Part model, mm, in its own coordinate system. A direction names the side the tool comes from. Round coordinates to 2 decimals unless told otherwise and drop trailing zeros. Write each loop counter-clockwise with the first axis right and the second up, starting at its lowest first coordinate (ties: lowest second). Pieces come first, ordered by that corner, then holes. Notation, with made-up numbers: M -20,41 L -11,41 A24 cw -11,74 Z; hole C 56,42.5 d1. An arc over 180 degrees is marked long. Answer as a JSON object with one key per item and string values. Group by question number.
1. Which spindle directions (+Z, -Z, +X, -X, +Y, -Y) get a long thin tool onto all of the face, cutting with end or side? Do faces 5 (the face through (3.631, 11.381, -16.235)), 6 (the face through (49.75, 2.6, -28.5)), 7 (the face through (53.76, 18.983, -40.521)), 8 (the face through (9.31, 18.15, -2.18)), 9 (the face through (29, 10, -7.62)). Say none if no direction does.
2. Drill centre lines: line 1 (Y direction, x = 53.5, z = -40.6); line 2 (X direction, y = 1.75, z = -35.5). Where is each one in solid material? Low to high. Write a range as from..to.
3. Band-saw the part on A-A, the plane z = -25. Write the cut outline in (x, y).
4. Two-plate mould, pull along Z, no slides. Class faces 1 (the face through (29, 10, -10.2)), 2 (the face through (4, 12, -39)), 3 (the face through (29, 3.65, -4)), 4 (the face through (4, 3, -31)): +Z half, -Z half, draft (parallel to the pull), parting line (faces both ways), or undercut.
5. Band-saw the part on C-C, the plane x = 53.5. Write the cut outline in (y, z), plus the area to 3 significant figures.
6. Band-saw the part on D-D, the plane y = 7. Write the cut outline in (x, z).
7. Drop flat-ended pins along their axis: pin 1 (1.5 mm diameter, centred on x = 46.5, y = 14.5, fed in from +Z); pin 2 (10 mm diameter, centred on x = 45, y = 12.5, fed in from -Z); pin 3 (6 mm diameter, centred on x = 35.5, y = 7.5, fed in from -Z); pin 4 (6 mm diameter, centred on x = 2.5, z = -32.5, fed in from +Y). Give the stop position or say it passes through.
8. Band-saw the part on B-B, the plane y = 9.75. Write the cut outline in (x, z), plus the area to 3 significant figures.
from build123d import *

# Parameters (mm, degrees)
SKETCH1_W                 = 57.5
SKETCH1_H                 = 42
BOSS_EXTRUDE1_DEPTH       = 20
CUT_EXTRUDE1_DEPTH        = 21
CUT_EXTRUDE2_DEPTH        = 58.5
CUT_EXTRUDE3_REACH        = 44
SKETCH4_R                 = 2
SKETCH5_W                 = 7.62
SKETCH5_H                 = 12.7
CUT_EXTRUDE4_DEPTH        = 58.5
M4X0_7_TAPPED_HOLE1_D     = 3.3
M4X0_7_TAPPED_HOLE1_DEPTH = 3.65
CHAMFER1_SIZE             = 3


with BuildPart() as part:
    # Sketch1 → Boss-Extrude1 (new body)
    with BuildSketch(Plane(origin=(0, 0, 0), x_dir=(1, 0, 0), z_dir=(0, 1, 0))):
        with Locations((28.75, 21)):
            Rectangle(SKETCH1_W, SKETCH1_H)
    extrude(amount=BOSS_EXTRUDE1_DEPTH)

    # Sketch2 → Cut-Extrude1 (cut, through all)
    with BuildSketch(Plane(origin=(0, 20, 0), x_dir=(1, 0, 0), z_dir=(0, 1, 0))):
        with BuildLine():
            Line((7.75, 42), (7.75, 15.2))
            ThreePointArc((7.75, 15.2), (9.214466094, 11.664466094), (12.75, 10.2))
            Line((12.75, 10.2), (44.75, 10.2))
            ThreePointArc((44.75, 10.2), (48.285533906, 11.664466094), (49.75, 15.2))
            Line((49.75, 15.2), (49.75, 42))
            Line((49.75, 42), (7.75, 42))
        make_face()
    extrude(amount=-CUT_EXTRUDE1_DEPTH, mode=Mode.SUBTRACT)

    # Sketch3 → Cut-Extrude2 (cut, through all)
    with BuildSketch(Plane(origin=(57.5, 0, 0), x_dir=(0, 0, -1), z_dir=(1, 0, 0))):
        Polygon((39, 20), (39, 3), (22.10352815, 3), (10.2, 20), align=None)
    extrude(amount=-CUT_EXTRUDE2_DEPTH, mode=Mode.SUBTRACT)

    # Sketch4 → Cut-Extrude3 (cut, up to next)
    with BuildSketch(Plane(origin=(0, 0, -42), x_dir=(-1, 0, 0), z_dir=(0, 0, -1)), mode=Mode.PRIVATE) as cut_extrude3_sk1:
        with Locations((-53.5, 17)):
            Circle(SKETCH4_R)
    cut_extrude3_tool1 = extrude(cut_extrude3_sk1.sketch, amount=-CUT_EXTRUDE3_REACH, mode=Mode.PRIVATE) & part.part
    add(cut_extrude3_tool1.solids().sort_by_distance((53.5, 17, -42))[0], mode=Mode.SUBTRACT)
    # Sketch4 → Cut-Extrude3 (cut, up to next)
    with BuildSketch(Plane(origin=(0, 0, -42), x_dir=(-1, 0, 0), z_dir=(0, 0, -1)), mode=Mode.PRIVATE) as cut_extrude3_sk2:
        with Locations((-4, 17)):
            Circle(SKETCH4_R)
    cut_extrude3_tool2 = extrude(cut_extrude3_sk2.sketch, amount=-CUT_EXTRUDE3_REACH, mode=Mode.PRIVATE) & part.part
    add(cut_extrude3_tool2.solids().sort_by_distance((4, 17, -42))[0], mode=Mode.SUBTRACT)
    # Sketch4 → Cut-Extrude3 (cut, up to next)
    with BuildSketch(Plane(origin=(0, 0, -42), x_dir=(-1, 0, 0), z_dir=(0, 0, -1)), mode=Mode.PRIVATE) as cut_extrude3_sk3:
        with Locations((-4, 7)):
            Circle(SKETCH4_R)
    cut_extrude3_tool3 = extrude(cut_extrude3_sk3.sketch, amount=-CUT_EXTRUDE3_REACH, mode=Mode.PRIVATE) & part.part
    add(cut_extrude3_tool3.solids().sort_by_distance((4, 7, -42))[0], mode=Mode.SUBTRACT)
    # Sketch4 → Cut-Extrude3 (cut, up to next)
    with BuildSketch(Plane(origin=(0, 0, -42), x_dir=(-1, 0, 0), z_dir=(0, 0, -1)), mode=Mode.PRIVATE) as cut_extrude3_sk4:
        with Locations((-53.5, 7)):
            Circle(SKETCH4_R)
    cut_extrude3_tool4 = extrude(cut_extrude3_sk4.sketch, amount=-CUT_EXTRUDE3_REACH, mode=Mode.PRIVATE) & part.part
    add(cut_extrude3_tool4.solids().sort_by_distance((53.5, 7, -42))[0], mode=Mode.SUBTRACT)

    # Sketch5 → Cut-Extrude4 (cut, through all)
    with BuildSketch(Plane(origin=(57.5, 0, 0), x_dir=(0, 0, -1), z_dir=(1, 0, 0))):
        with Locations((3.81, 10)):
            Rectangle(SKETCH5_W, SKETCH5_H)
    extrude(amount=-CUT_EXTRUDE4_DEPTH, mode=Mode.SUBTRACT)

    # M4x0.7 Tapped Hole1
    with Locations(Plane(origin=(0, 20, 0), x_dir=(1, 0, 0), z_dir=(0, 1, 0))):
        with Locations((8, 3.18), (21.833333333, 3.18), (35.666666667, 3.18), (49.5, 3.18)):
            Hole(M4X0_7_TAPPED_HOLE1_D / 2, depth=M4X0_7_TAPPED_HOLE1_DEPTH)

    # Chamfer1
    chamfer1_edges = [part.edges().sort_by_distance(p)[0] for p in [
        (28.75, 0, 0),
    ]]
    chamfer(chamfer1_edges, length=CHAMFER1_SIZE)


solid = part.part
Worked answers:
{
 "1": {"face 5": "+X, -X, +Y", "face 6": "-Z, +Y, -Y", "face 7": "-Z", "face 8": "+Y", "face 9": "+Z, +X, -X"},
 "2": {"line 1": "y = 0..5, 9..15, 19..20", "line 2": "x = 0..7.75, 49.75..57.5"},
 "3": {"outline": "M 0,0 L 7.75,0 L 7.75,3 L 0,3 Z; M 49.75,0 L 57.5,0 L 57.5,3 L 49.75,3 Z"},
 "4": {"face 1": "-Z half", "face 2": "undercut", "face 3": "draft", "face 4": "undercut"},
 "5": {"outline": "M 0,-42 L 5,-42 L 5,-39 L 3,-39 L 3,-22.1 L 20,-10.2 L 20,0 L 16.35,0 L 16.35,-7.62 L 3.65,-7.62 L 3.65,0 L 3,0 L 0,-3 Z; M 9,-42 L 15,-42 L 15,-39 L 9,-39 Z; M 19,-42 L 20,-42 L 20,-39 L 19,-39 Z", "area": "326 mm^2"},
 "6": {"outline": "M 0,-42 L 2,-42 L 2,-39 L 0,-39 Z; M 0,-19.3 L 7.75,-19.3 L 7.75,-15.2 A5 cw 12.75,-10.2 L 44.75,-10.2 A5 cw 49.75,-15.2 L 49.75,-19.3 L 57.5,-19.3 L 57.5,-7.62 L 0,-7.62 Z; M 6,-42 L 7.75,-42 L 7.75,-39 L 6,-39 Z; M 49.75,-42 L 51.5,-42 L 51.5,-39 L 49.75,-39 Z; M 55.5,-42 L 57.5,-42 L 57.5,-39 L 55.5,-39 Z"},
 "7": {"pin 1": "stops at z = -7.62", "pin 2": "stops at z = -42", "pin 3": "stops at z = -10.2", "pin 4": "stops at y = 3"},
 "8": {"outline": "M 0,-42 L 7.75,-42 L 7.75,-39 L 0,-39 Z; M 0,-17.38 L 7.75,-17.38 L 7.75,-15.2 A5 cw 12.75,-10.2 L 44.75,-10.2 A5 cw 49.75,-15.2 L 49.75,-17.38 L 57.5,-17.38 L 57.5,-7.62 L 0,-7.62 Z; M 49.75,-42 L 57.5,-42 L 57.5,-39 L 49.75,-39 Z", "area": "317 mm^2"}
}
